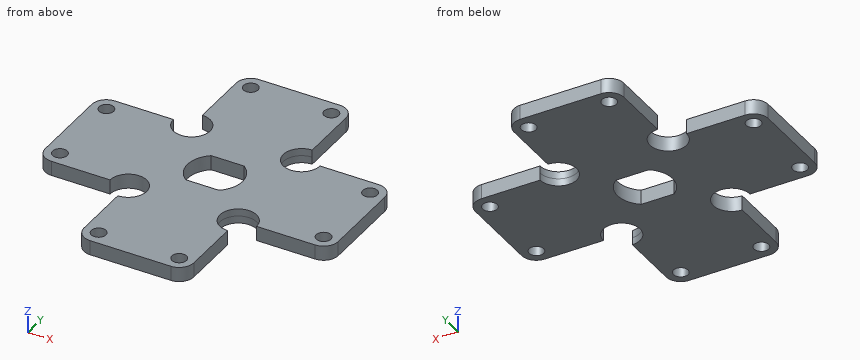
```python
from build123d import *

# Parameters (mm, degrees)
F1_R          = 2
F3_DEPTH      = 2
F4_DEPTH      = 2.001
F4_DEPTH_BACK = 2.001
F2_R          = 5
F5_DEPTH      = 2.001
F5_DEPTH_BACK = 2.001


with BuildPart() as f3:
    # F1 (on Top) → F3 (new body, symmetric)
    with BuildSketch(Plane.XY):
        with BuildLine():
            Line((-15, 36), (-15, 15))
            Line((-15, 15), (-36, 15))
            ThreePointArc((-36, 15), (-38.8284271247, 13.8284271247), (-40, 11))
            Line((-40, 11), (-40, 0))
            Line((-40, 0), (-40, -11))
            ThreePointArc((-40, -11), (-38.8284271247, -13.8284271247), (-36, -15))
            Line((-36, -15), (-15, -15))
            Line((-15, -15), (-15, -36))
            ThreePointArc((-15, -36), (-13.8284271247, -38.8284271247), (-11, -40))
            Line((-11, -40), (0, -40))
            Line((0, -40), (11, -40))
            ThreePointArc((11, -40), (13.8284271247, -38.8284271247), (15, -36))
            Line((15, -36), (15, -15))
            Line((15, -15), (36, -15))
            ThreePointArc((36, -15), (38.8284271247, -13.8284271247), (40, -11))
            Line((40, -11), (40, 0))
            Line((40, 0), (40, 11))
            ThreePointArc((40, 11), (38.8284271247, 13.8284271247), (36, 15))
            Line((36, 15), (15, 15))
            Line((15, 15), (15, 36))
            ThreePointArc((15, 36), (13.8284271247, 38.8284271247), (11, 40))
            Line((11, 40), (0, 40))
            Line((0, 40), (-11, 40))
            ThreePointArc((-11, 40), (-13.8284271247, 38.8284271247), (-15, 36))
        make_face()
        with Locations((-11, -36)):
            Circle(F1_R, mode=Mode.SUBTRACT)
        with Locations((-36, -11)):
            Circle(F1_R, mode=Mode.SUBTRACT)
        with Locations((11, -36)):
            Circle(F1_R, mode=Mode.SUBTRACT)
        with Locations((36, -11)):
            Circle(F1_R, mode=Mode.SUBTRACT)
        with Locations((-36, 11)):
            Circle(F1_R, mode=Mode.SUBTRACT)
        with Locations((-11, 36)):
            Circle(F1_R, mode=Mode.SUBTRACT)
        with Locations((36, 11)):
            Circle(F1_R, mode=Mode.SUBTRACT)
        with Locations((11, 36)):
            Circle(F1_R, mode=Mode.SUBTRACT)
    extrude(amount=F3_DEPTH, both=True)

    # F0 (on Top) → F4 (cut, two sides)
    with BuildSketch(Plane.XY) as f4_sk:
        with BuildLine():
            Line((4.5, 6), (-4.5, 6))
            ThreePointArc((-4.5, 6), (-7.5, 0), (-4.5, -6))
            Line((-4.5, -6), (4.5, -6))
            ThreePointArc((4.5, -6), (7.5, 0), (4.5, 6))
        make_face()
    extrude(amount=-F4_DEPTH, mode=Mode.SUBTRACT)
    extrude(f4_sk.sketch, amount=F4_DEPTH_BACK, mode=Mode.SUBTRACT)

    # F2 (on Top) → F5 (cut, two sides)
    with BuildSketch(Plane.XY) as f5_sk:
        with Locations((-15, 15)):
            Circle(F2_R)
        with Locations((-15, -15)):
            Circle(F2_R)
        with Locations((15, -15)):
            Circle(F2_R)
        with Locations((15, 15)):
            Circle(F2_R)
    extrude(amount=-F5_DEPTH, mode=Mode.SUBTRACT)
    extrude(f5_sk.sketch, amount=F5_DEPTH_BACK, mode=Mode.SUBTRACT)


solid = f3.part
```
Check sheet for the modelled part. Datum: model origin and axes. Units: mm. Coordinates: 2 decimals unless noted, no trailing zeros. Write each loop counter-clockwise with the first axis right and the second up, starting at its lowest first coordinate (ties: lowest second). Pieces come first, ordered by that corner, then holes. Notation, with made-up numbers: M -30.75,65.5 L -14.75,65.5 A17 ccw -14.75,88.5 Z; hole C 88,82.5 d6. An arc over 180 degrees is marked long. Use one line per item in the form item = value.
Item 1: Gauge pin test, flat end, axial feed: pin 1 Ø1.2 at (x, z) = (-24.5, 1) entering from -Y. Record the tip position at first contact, or that the pin passes through.
Answer below:
pin_1 = -15
Item 2: Sectioned sample at C-C, the plane x = 12. Record the cut outline in (y, z).
Answer below:
outline = M -39.87,-2 L -37.73,-2 L -37.73,2 L -39.87,2 Z; M -34.27,-2 L -19,-2 L -19,2 L -34.27,2 Z; M -11,-2 L 11,-2 L 11,2 L -11,2 Z; M 19,-2 L 34.27,-2 L 34.27,2 L 19,2 Z; M 37.73,-2 L 39.87,-2 L 39.87,2 L 37.73,2 Z
Item 3: Sectioned sample at D-D, the plane z = -1. State how many separate pieces and enclosed holes the cut face has, and give its area (3 significant figures).
Answer below:
separate_pieces = 1
enclosed_holes = 9
area = 3,380 mm^2
Item 4: Material ranges on L1, parallel to Y at x = -36, z = -1.1; L2, parallel to X at y = -14.5, z = 0.75; L3, parallel to Y at x = 28, z = 0.65, recorded low to high. Write a range as from..to.
Answer below:
L1 = -15..-13, -9..9, 13..15
L2 = -37.94..-19.97, -10.03..10.03, 19.97..37.94
L3 = -15..15
Item 5: Sectioned sample at B-B, the plane y = 1.5. Record the cut outline in (x, z).
Answer below:
outline = M -40,-2 L -7.35,-2 L -7.35,2 L -40,2 Z; M 7.35,-2 L 40,-2 L 40,2 L 7.35,2 Z
Item 6: Sectioned sample at A-A, the plane x = -2.5. Record the cut outline in (y, z), and give its area (3 significant figures).
Answer below:
outline = M -40,-2 L -6,-2 L -6,2 L -40,2 Z; M 6,-2 L 40,-2 L 40,2 L 6,2 Z
area = 272 mm^2
